Could you check a few things on this model? Use its own coordinates, in mm. Give positions to 0.01 mm unless a question says otherwise; leave off trailing zeros. Loops run counter-clockwise (first coordinate to the right, second up) from the corner with the lowest first, then second, coordinate; pieces in that order, holes last. Notation, with made-up numbers: (-11, 87) -> (2, 87) arc R32 cw to (2, 121) -> close; hole circle Ø4 at (44, -30). An arc over 180 degrees is marked (long way). Write each question's results on one line, items separated by ' | '. Start each with the question number.
Q1. Will these pins go through, and if not, where does the flat tip stop? P1, Ø1.8, axis at x = -24, y = 1, coming from the +Z side; P2, Ø4.5, axis at y = 0, z = 0, coming from the -X side; P3, Ø5, axis at x = -33, z = -0.5, coming from the +Y side.
Q2. If I drill on line 1 along Y through (x, z) = (29, 0); line 2 along Z through (x, y) = (40, 8.5); line 3 along Z through (x, y) = (-23.5, -3), over which ranges is the centre line in solid material (lowest first)?
Q3. If we section it at A-A, the plane z = 0: List the corners of the cut face in (x, y) for me.
from build123d import *

# Parameters (mm, degrees)
SKETCH1_R           = 2.5
BOSS_EXTRUDE2_DEPTH = 66.25


with BuildPart() as part:
    # Sketch1 → Boss-Extrude2 (new, symmetric)
    with BuildSketch(Plane(origin=(0, 0, 0), x_dir=(0, 0, -1), z_dir=(1, 0, 0))):
        with BuildLine():
            Line((10, 4.2), (10, 8.5))
            ThreePointArc((10, 8.5), (9.560660172, 9.560660172), (8.5, 10))
            Line((8.5, 10), (4.2, 10))
            ThreePointArc((4.2, 10), (3.987867966, 9.912132034), (3.9, 9.7))
            Line((3.9, 9.7), (3.9, 9.5))
            ThreePointArc((3.9, 9.5), (3.812132034, 9.287867966), (3.6, 9.2))
            Line((3.6, 9.2), (3.4, 9.2))
            ThreePointArc((3.4, 9.2), (3.187867966, 9.112132034), (3.1, 8.9))
            Line((3.1, 8.9), (3.1, 8.5))
            ThreePointArc((3.1, 8.5), (3.187867966, 8.287867966), (3.4, 8.2))
            Line((3.4, 8.2), (5.2, 8.2))
            ThreePointArc((5.2, 8.2), (5.412132034, 8.112132034), (5.5, 7.9))
            Line((5.5, 7.9), (5.5, 6.521320344))
            Line((5.5, 6.521320344), (4.118019485, 5.139339828))
            ThreePointArc((4.118019485, 5.139339828), (3.631384461, 4.814180701), (3.057359313, 4.7))
            Line((3.057359313, 4.7), (-3.057359313, 4.7))
            ThreePointArc((-3.057359313, 4.7), (-3.631384461, 4.814180701), (-4.118019485, 5.139339828))
            Line((-4.118019485, 5.139339828), (-5.5, 6.521320344))
            Line((-5.5, 6.521320344), (-5.5, 7.9))
            ThreePointArc((-5.5, 7.9), (-5.412132034, 8.112132034), (-5.2, 8.2))
            Line((-5.2, 8.2), (-3.4, 8.2))
            ThreePointArc((-3.4, 8.2), (-3.187867966, 8.287867966), (-3.1, 8.5))
            Line((-3.1, 8.5), (-3.1, 8.9))
            ThreePointArc((-3.1, 8.9), (-3.187867966, 9.112132034), (-3.4, 9.2))
            Line((-3.4, 9.2), (-3.6, 9.2))
            ThreePointArc((-3.6, 9.2), (-3.812132034, 9.287867966), (-3.9, 9.5))
            Line((-3.9, 9.5), (-3.9, 9.7))
            ThreePointArc((-3.9, 9.7), (-3.987867966, 9.912132034), (-4.2, 10))
            Line((-4.2, 10), (-8.5, 10))
            ThreePointArc((-8.5, 10), (-9.560660172, 9.560660172), (-10, 8.5))
            Line((-10, 8.5), (-10, 4.2))
            ThreePointArc((-10, 4.2), (-9.912132034, 3.987867966), (-9.7, 3.9))
            Line((-9.7, 3.9), (-9.5, 3.9))
            ThreePointArc((-9.5, 3.9), (-9.287867966, 3.812132034), (-9.2, 3.6))
            Line((-9.2, 3.6), (-9.2, 3.4))
            ThreePointArc((-9.2, 3.4), (-9.112132034, 3.187867966), (-8.9, 3.1))
            Line((-8.9, 3.1), (-8.5, 3.1))
            ThreePointArc((-8.5, 3.1), (-8.287867966, 3.187867966), (-8.2, 3.4))
            Line((-8.2, 3.4), (-8.2, 5.2))
            ThreePointArc((-8.2, 5.2), (-8.112132034, 5.412132034), (-7.9, 5.5))
            Line((-7.9, 5.5), (-6.6, 5.5))
            Line((-6.6, 5.5), (-5.139339828, 4.039339828))
            ThreePointArc((-5.139339828, 4.039339828), (-4.814180701, 3.552704805), (-4.7, 2.978679656))
            Line((-4.7, 2.978679656), (-4.7, -2.978679656))
            ThreePointArc((-4.7, -2.978679656), (-4.814180701, -3.552704805), (-5.139339828, -4.039339828))
            Line((-5.139339828, -4.039339828), (-6.6, -5.5))
            Line((-6.6, -5.5), (-7.9, -5.5))
            ThreePointArc((-7.9, -5.5), (-8.112132034, -5.412132034), (-8.2, -5.2))
            Line((-8.2, -5.2), (-8.2, -3.4))
            ThreePointArc((-8.2, -3.4), (-8.287867966, -3.187867966), (-8.5, -3.1))
            Line((-8.5, -3.1), (-8.9, -3.1))
            ThreePointArc((-8.9, -3.1), (-9.112132034, -3.187867966), (-9.2, -3.4))
            Line((-9.2, -3.4), (-9.2, -3.6))
            ThreePointArc((-9.2, -3.6), (-9.287867966, -3.812132034), (-9.5, -3.9))
            Line((-9.5, -3.9), (-9.7, -3.9))
            ThreePointArc((-9.7, -3.9), (-9.912132034, -3.987867966), (-10, -4.2))
            Line((-10, -4.2), (-10, -8.5))
            ThreePointArc((-10, -8.5), (-9.560660172, -9.560660172), (-8.5, -10))
            Line((-8.5, -10), (-4.2, -10))
            ThreePointArc((-4.2, -10), (-3.987867966, -9.912132034), (-3.9, -9.7))
            Line((-3.9, -9.7), (-3.9, -9.5))
            ThreePointArc((-3.9, -9.5), (-3.812132034, -9.287867966), (-3.6, -9.2))
            Line((-3.6, -9.2), (-3.4, -9.2))
            ThreePointArc((-3.4, -9.2), (-3.187867966, -9.112132034), (-3.1, -8.9))
            Line((-3.1, -8.9), (-3.1, -8.5))
            ThreePointArc((-3.1, -8.5), (-3.187867966, -8.287867966), (-3.4, -8.2))
            Line((-3.4, -8.2), (-5.2, -8.2))
            ThreePointArc((-5.2, -8.2), (-5.412132034, -8.112132034), (-5.5, -7.9))
            Line((-5.5, -7.9), (-5.5, -6.521320344))
            Line((-5.5, -6.521320344), (-4.118019485, -5.139339828))
            ThreePointArc((-4.118019485, -5.139339828), (-3.631384461, -4.814180701), (-3.057359313, -4.7))
            Line((-3.057359313, -4.7), (3.057359313, -4.7))
            ThreePointArc((3.057359313, -4.7), (3.631384461, -4.814180701), (4.118019485, -5.139339828))
            Line((4.118019485, -5.139339828), (5.5, -6.521320344))
            Line((5.5, -6.521320344), (5.5, -7.9))
            ThreePointArc((5.5, -7.9), (5.412132034, -8.112132034), (5.2, -8.2))
            Line((5.2, -8.2), (3.4, -8.2))
            ThreePointArc((3.4, -8.2), (3.187867966, -8.287867966), (3.1, -8.5))
            Line((3.1, -8.5), (3.1, -8.9))
            ThreePointArc((3.1, -8.9), (3.187867966, -9.112132034), (3.4, -9.2))
            Line((3.4, -9.2), (3.6, -9.2))
            ThreePointArc((3.6, -9.2), (3.812132034, -9.287867966), (3.9, -9.5))
            Line((3.9, -9.5), (3.9, -9.7))
            ThreePointArc((3.9, -9.7), (3.987867966, -9.912132034), (4.2, -10))
            Line((4.2, -10), (8.5, -10))
            ThreePointArc((8.5, -10), (9.560660172, -9.560660172), (10, -8.5))
            Line((10, -8.5), (10, -4.2))
            ThreePointArc((10, -4.2), (9.912132034, -3.987867966), (9.7, -3.9))
            Line((9.7, -3.9), (9.5, -3.9))
            ThreePointArc((9.5, -3.9), (9.287867966, -3.812132034), (9.2, -3.6))
            Line((9.2, -3.6), (9.2, -3.4))
            ThreePointArc((9.2, -3.4), (9.112132034, -3.187867966), (8.9, -3.1))
            Line((8.9, -3.1), (8.5, -3.1))
            ThreePointArc((8.5, -3.1), (8.287867966, -3.187867966), (8.2, -3.4))
            Line((8.2, -3.4), (8.2, -5.2))
            ThreePointArc((8.2, -5.2), (8.112132034, -5.412132034), (7.9, -5.5))
            Line((7.9, -5.5), (6.6, -5.5))
            Line((6.6, -5.5), (5.139339828, -4.039339828))
            ThreePointArc((5.139339828, -4.039339828), (4.814180701, -3.552704805), (4.7, -2.978679656))
            Line((4.7, -2.978679656), (4.7, 2.978679656))
            ThreePointArc((4.7, 2.978679656), (4.814180701, 3.552704805), (5.139339828, 4.039339828))
            Line((5.139339828, 4.039339828), (6.6, 5.5))
            Line((6.6, 5.5), (7.9, 5.5))
            ThreePointArc((7.9, 5.5), (8.112132034, 5.412132034), (8.2, 5.2))
            Line((8.2, 5.2), (8.2, 3.4))
            ThreePointArc((8.2, 3.4), (8.287867966, 3.187867966), (8.5, 3.1))
            Line((8.5, 3.1), (8.9, 3.1))
            ThreePointArc((8.9, 3.1), (9.112132034, 3.187867966), (9.2, 3.4))
            Line((9.2, 3.4), (9.2, 3.6))
            ThreePointArc((9.2, 3.6), (9.287867966, 3.812132034), (9.5, 3.9))
            Line((9.5, 3.9), (9.7, 3.9))
            ThreePointArc((9.7, 3.9), (9.912132034, 3.987867966), (10, 4.2))
        make_face()
        Circle(SKETCH1_R, mode=Mode.SUBTRACT)
    extrude(amount=BOSS_EXTRUDE2_DEPTH, both=True)


solid = part.part
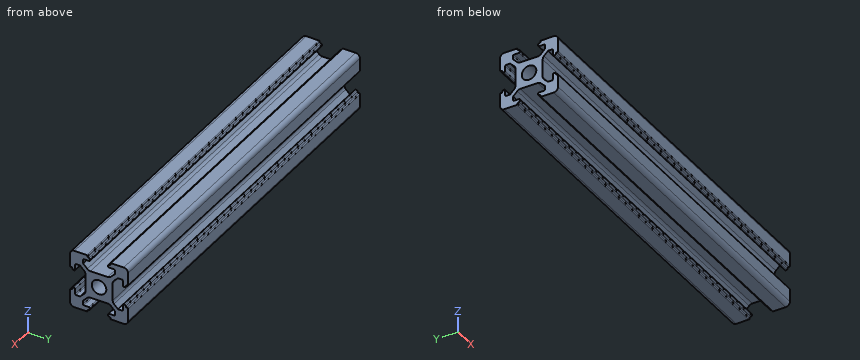
Final values:
1) P1: stops at z = 4.7 | P2: passes through | P3: stops at y = 4.7
2) line 1: y = -4.7 to -2.5, 2.5 to 4.7 | line 2: z = -10 to -3.1, 3.1 to 10 | line 3: z = -4.7 to 4.7
3) outline: (-66.25, -4.7) -> (66.25, -4.7) -> (66.25, -2.5) -> (-66.25, -2.5) -> close; (-66.25, 2.5) -> (66.25, 2.5) -> (66.25, 4.7) -> (-66.25, 4.7) -> close
